from build123d import *

# Parameters (mm, degrees)
BOSS_EXTRUDE1_DEPTH = 15
CUT_EXTRUDE1_REACH  = 15.469
SKETCH2_R           = 2.5


with BuildPart() as part:
    # Sketch1 → Boss-Extrude1 (new body)
    with BuildSketch(Plane.XY):
        with BuildLine():
            Line((0, 0), (0, 6.5))
            ThreePointArc((0, 6.5), (10.284515004, 50.25), (0, 94))
            Line((0, 94), (0, 100.5))
            ThreePointArc((0, 100.5), (13.469469939, 50.25), (0, 0))
        make_face()
    extrude(amount=BOSS_EXTRUDE1_DEPTH)

    # Sketch2 → Cut-Extrude1 (cut, up to next)
    with BuildSketch(Plane.ZY, mode=Mode.PRIVATE) as cut_extrude1_sk1:
        with Locations((7.5, 97.25)):
            Circle(SKETCH2_R)
    cut_extrude1_tool1 = extrude(cut_extrude1_sk1.sketch, amount=-CUT_EXTRUDE1_REACH, mode=Mode.PRIVATE) & part.part
    add(cut_extrude1_tool1.solids().sort_by_distance((0, 97.25, 7.5))[0], mode=Mode.SUBTRACT)
    # Sketch2 → Cut-Extrude1 (cut, up to next)
    with BuildSketch(Plane.ZY, mode=Mode.PRIVATE) as cut_extrude1_sk2:
        with Locations((7.5, 3.25)):
            Circle(SKETCH2_R)
    cut_extrude1_tool2 = extrude(cut_extrude1_sk2.sketch, amount=-CUT_EXTRUDE1_REACH, mode=Mode.PRIVATE) & part.part
    add(cut_extrude1_tool2.solids().sort_by_distance((0, 3.25, 7.5))[0], mode=Mode.SUBTRACT)


solid = part.part
Design review of the part built by this model. Coordinates are the model's own, in mm. Round coordinates to 2 decimals unless told otherwise and drop trailing zeros. Loops run counter-clockwise (first coordinate to the right, second up) from the corner with the lowest first, then second, coordinate; pieces in that order, holes last. Notation, with made-up numbers: M -16,43.25 L 18,43.25 A13 ccw 18,48.25 Z; hole C 26,73 d5. An arc over 180 degrees is marked long. Answer as a JSON object with one key per item and string values.
Item 1: Wall thickness on L1, parallel to Z at x = 0.9, y = 97.25; L2, parallel to Y at x = 2.3, z = 7.5; L3, parallel to Y at x = 2.45, z = 7.5: over which ranges is each line inside the solid? List them lowest first. Write a range as from..to.
Answer sheet:
{"L1": "z = 0..5, 10..15", "L2": "y = 5.75..11.46, 89.04..94.75", "L3": "y = 5.75..11.81, 88.69..94.75"}
Item 2: Clearance check with flat-ended pins moving along their axes: P1, Ø1.5, axis at x = 2, z = 13, coming from the -Y side; P2, Ø4, axis at y = 52.5, z = 4.5, coming from the +X side; P3, Ø6.5, axis at y = 3.25, z = 7.5, coming from the +X side. State where each tip first meets the part, or that it passes through.
Answer sheet:
{"P1": "stops at y = 2.23", "P2": "stops at x = 13.47", "P3": "stops at x = 3.44"}
Item 3: We need section D-D on z = 2.25. Give the boundary of the cut face in (x, y).
Answer sheet:
{"outline": "M 0,0 A100.47 ccw 0,100.5 L 0,94 A98.2 cw 0,6.5 Z"}
Item 4: We need section C-C on y = 97.25. Give the boundary of the cut face in (x, z).
Answer sheet:
{"outline": "M 0,0 L 1.8,0 L 1.8,5 L 0,5 Z; M 0,10 L 1.8,10 L 1.8,15 L 0,15 Z"}
Item 5: We need section B-B on x = 9. Give the boundary of the cut face in (y, z).
Answer sheet:
{"outline": "M 20.62,0 L 34.42,0 L 34.42,15 L 20.62,15 Z; M 66.08,0 L 79.88,0 L 79.88,15 L 66.08,15 Z"}
Item 6: We need section A-A on z = 6.25. Give the boundary of the cut face in (x, y).
Answer sheet:
{"outline": "M 0,0 A100.47 ccw 0.62,1.08 L 0,1.08 Z; M 0,5.42 L 2.91,5.42 A100.47 ccw 2.91,95.08 L 0,95.08 L 0,94 A98.2 cw 0,6.5 Z; M 0,99.42 L 0.62,99.42 A100.47 ccw 0,100.5 Z"}
Item 7: The part is to be moulded in two halves that separate along Z. For faces 1 (the cylindrical face through (1.17, 5.73, 7.17)), 2 (the flat face through (12, 50, 0)), 3 (the flat face through (0, 1, 9)), 4 (the flat face through (12, 50, 15)), say which applies: pulls with the +Z half, pulls with the -Z half, needs draft (parallel to the pull), parting line crosses it, or undercut.
Answer sheet:
{"face 1": "undercut", "face 2": "pulls with the -Z half", "face 3": "needs draft", "face 4": "pulls with the +Z half"}
